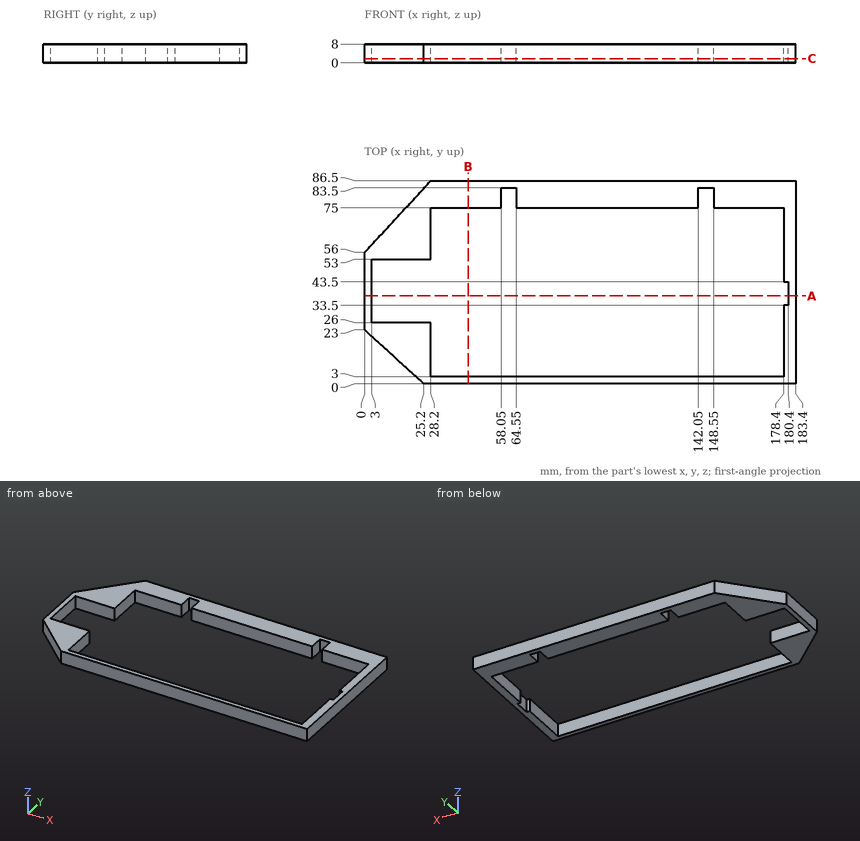
The drawing under review shows one solid part. Ordinate dimensions are in mm from its lowest x, y, z. Round coordinates to 2 decimals unless told otherwise and drop trailing zeros. Loops run counter-clockwise (first coordinate to the right, second up) from the corner with the lowest first, then second, coordinate; pieces in that order, holes last. Notation, with made-up numbers: (35, 75) - (75, 75) arc R34 ccw to (75, 111) - close; hole circle Ø11 at (-28.5, 63.5). An arc over 180 degrees is marked (long way). Use one line per item in the form item = value.
Item 1: For line 1 (Y direction, x = 76, z = 6); line 2 (X direction, y = 38, z = 6.75); line 3 (X direction, y = 78.5, z = 2.25), list the stretches that pass through material, from the lowest coordinate up.
Answers:
line_1 = 0 to 3, 75 to 86.5
line_2 = 0 to 3, 180.4 to 183.4
line_3 = 20.8 to 58.05, 64.55 to 142.05, 148.55 to 183.4
Item 2: Consider section B-B on x = 44. Write out the cut boundary in (y, z), then the cut area to 3 significant figures.
Answers:
outline = (0, 0) - (3, 0) - (3, 8) - (0, 8) - close; (75, 0) - (86.5, 0) - (86.5, 8) - (75, 8) - close
area = 116 mm^2
Item 3: Consider section C-C on z = 1.75. Write out the cut boundary in (x, y).
Answers:
outline = (0, 23) - (25.2, 0) - (183.4, 0) - (183.4, 86.5) - (28.2, 86.5) - (0, 56) - close; hole (3, 26) - (28.2, 26) - (28.2, 3) - (178.4, 3) - (178.4, 33.5) - (180.4, 33.5) - (180.4, 43.5) - (178.4, 43.5) - (178.4, 75) - (148.55, 75) - (148.55, 83.5) - (142.05, 83.5) - (142.05, 75) - (64.55, 75) - (64.55, 83.5) - (58.05, 83.5) - (58.05, 75) - (28.2, 75) - (28.2, 53) - (3, 53) - close
Item 4: Consider section A-A on y = 37.5. Write out the cut boundary in (x, z), then the cut area to 3 significant figures.
Answers:
outline = (0, 0) - (3, 0) - (3, 8) - (0, 8) - close; (180.4, 0) - (183.4, 0) - (183.4, 8) - (180.4, 8) - close
area = 48.0 mm^2
Item 5: Clearance check with flat-ended pins moving along their axes: P1, Ø4, axis at y = 80, z = 4, coming from the -X side; P2, Ø4, axis at x = 13, z = 5, coming from the +Y side; P3, Ø4, axis at y = 64, z = 1.5, coming from the -X side; P4, Ø2, axis at x = 137.5, y = 72.5, coming from the +Z side. State where each tip first meets the part, or that it passes through.
Answers:
P1 = 20.34
P2 = 72.22
P3 = 5.55
P4 = through
